For this review, take the finished solid that the model builds, in its own axes (mm). A direction names the side the tool comes from. Coordinates: 2 decimals unless noted, no trailing zeros. Loops run counter-clockwise (first coordinate to the right, second up) from the corner with the lowest first, then second, coordinate; pieces in that order, holes last. Notation, with made-up numbers: M 60,72 L 65,72 A24 ccw 65,101 Z; hole C -12.75,11.5 d5. An arc over 180 degrees is marked long. Answer as a JSON object with one key per item and string values. Group by question number.
Item 1: Insertion check: pin 1 (1 mm diameter, centred on y = 271, z = 5, fed in from +X); pin 2 (4 mm diameter, centred on x = 8.26, y = 258.75, fed in from -Z); pin 3 (1 mm diameter, centred on x = 10.5, z = 1, fed in from -Y) (3 decimals); pin 4 (5 mm diameter, centred on x = -8.26, y = 287.35, fed in from +Z). Each pin has a flat end and moves straight along its axis. Give the tip position at first contact, or say it passes through.
Item 2: Tool access review of faces 4 (the face through (4.5, 273.2, 4.475)), 5 (the face through (-16.783, 270.968, 3.145)): name each direction out of +Z, -Z, +X, -X, +Y, -Y from which nothing blocks a thin tool from reaching the whole face with its end or side.
Item 3: Add section D-D (x = -16.51). State the section outline as (y, z) points (3 decimals), then the cut area to 3 significant figures.
Item 4: Add section C-C (z = 2). State the section outline as (x, y) points (3 decimals), then the cut area to 3 significant figures.
Item 5: Mouldability with a two-part tool opening along Y and no side actions: class faces 1 (the face through (-2.401, 283.863, 1.893)), 2 (the face through (0, 278, 7.015)), 3 (the face through (-4.543, 293.507, 3.458)) as +Y half, -Y half, draft (parallel to the pull), parting line (faces both ways), or undercut.
Item 6: Add section A-A (x = 0). State the section outline as (y, z) points (3 decimals).
Item 7: Add section B-B (y = 273.05). State the section outline as (x, z) points (3 decimals), then the cut area to 3 significant figures.
Item 8: Wall thickness on L1, parallel to Y at x = 0, z = 1.35 (3 decimals); L2, parallel to Y at x = 10, z = 6 (3 decimals); L3, parallel to Y at x = 8, z = 0.75: over which ranges is each line inside the solid? List them lowest first. Write a range as from..to.
Autodesk Inventor part; units mm, degrees
ref_plane "YZ Plane" through (0, 0, 0) normal (1, 0, 0) x (0, 1, 0)
ref_plane "XZ Plane" through (0, 0, 0) normal (0, 1, 0) x (-1, 0, 0)
ref_plane "XY Plane" through (0, 0, 0) normal (0, 0, 1) x (1, 0, 0)
sketch "Sketch1" plane through (0, 0, 0) normal (0, 0, 1) x (1, 0, 0)
  circle A0 centre (0, 273.05) radius 20.955
  circle A1 centre (0, 273.05) radius 11
  arc A2 (219.754, -304.8) -> (225.7704, -296.4188) centre (219.754, -298.45) ccw
  line L0 (225.7704, -296.4188) -> (30.0819, 283.206)
  arc A3 (30.0819, 283.206) -> (-30.0819, 283.206) centre (0, 273.05) ccw
  line L1 (-30.0819, 283.206) -> (-225.7704, -296.4188)
  arc A4 (-225.7704, -296.4188) -> (-219.754, -304.8) centre (-219.754, -298.45) ccw
  line L2 (-219.754, -304.8) -> (219.754, -304.8)
  line L3 (-38.1, -17.4222) -> (-38.1, -222.25)
  arc A5 (-44.45, -228.6) -> (-38.1, -222.25) centre (-44.45, -222.25) ccw
  line L4 (-44.45, -228.6) -> (-113.6024, -228.6)
  arc A6 (-119.6188, -220.2188) -> (-113.6024, -228.6) centre (-113.6024, -222.25) ccw
  line L5 (-119.6188, -220.2188) -> (-50.4664, -15.391)
  arc A7 (-38.1, -17.4222) -> (-50.4664, -15.391) centre (-44.45, -17.4222) ccw
  line L6 (113.6024, -228.6) -> (44.45, -228.6)
  arc A8 (38.1, -222.25) -> (44.45, -228.6) centre (44.45, -222.25) ccw
  line L7 (38.1, -222.25) -> (38.1, -17.4222)
  arc A9 (50.4664, -15.391) -> (38.1, -17.4222) centre (44.45, -17.4222) ccw
  line L8 (50.4664, -15.391) -> (119.6188, -220.2188)
  arc A10 (113.6024, -228.6) -> (119.6188, -220.2188) centre (113.6024, -222.25) ccw
  circle A11 centre (-204.2059, -292.1) radius 2
  circle A12 centre (-187.0552, -241.3) radius 2
  circle A13 centre (187.0552, -241.3) radius 2
  circle A14 centre (204.2059, -292.1) radius 2
  circle A15 centre (19.05, -241.3) radius 2
  circle A16 centre (19.05, -292.1) radius 2
  circle A17 centre (-19.05, -292.1) radius 2
  circle A18 centre (-19.05, -241.3) radius 2
  circle A19 centre (8.255, 287.3481) radius 2
  circle A20 centre (-8.255, 287.3481) radius 2
  circle A21 centre (-16.51, 273.05) radius 2
  circle A22 centre (-8.255, 258.7519) radius 2
  circle A23 centre (8.255, 258.7519) radius 2
  circle A24 centre (16.51, 273.05) radius 2
  circle A25 centre (0, 273.05) radius 11
  circle A26 centre (0, 273.05) radius 11.0762
  circle A27 centre (-8.255, 287.3481) radius 2.1
  circle A28 centre (8.255, 287.3481) radius 2.1
  circle A29 centre (16.51, 273.05) radius 2.1
  circle A30 centre (8.255, 258.7519) radius 2.1
  circle A31 centre (-8.255, 258.7519) radius 2.1
  circle A32 centre (-16.51, 273.05) radius 2.1
  circle A33 centre (0, 273.05) radius 4.35
  point P0 (0, 0)
  dimension "d0" = 0.0762
  dimension "d1" = 4.2
  dimension "d2" = 4.2
  dimension "d3" = 4.2
  dimension "d4" = 4.2
  dimension "d5" = 4.2
  dimension "d6" = 4.2
  dimension "d9" = 8.7
extrude "Extrusion1" add sketch "Sketch1" along normal blind 7.015 contours A0 | A1 | A26
extrude "Extrusion2" cut sketch "Sketch1" along normal blind 4.475 contours A1 | A26 | A33
chamfer "Chamfer1" distance 0.635 angle 45 7 edges at (-11.0762, 273.05, 4.475) (6.155, 287.3481, 7.015) (-10.355, 287.3481, 7.015) (-18.61, 273.05, 7.015) (-10.355, 258.7519, 7.015) (6.155, 258.7519, 7.015) (14.41, 273.05, 7.015)
properties part number "MainOuterBearingMount"
From the geometry:
{
 "1": {"pin 1": "stops at x = 20.9", "pin 2": "passes through", "pin 3": "stops at y = 254.635", "pin 4": "stops at z = 6.79"},
 "2": {"face 4": "-Z", "face 5": "+Z, -Z"},
 "3": {"outline": "M 260.145,0 L 270.95,0 L 270.95,6.38 L 270.315,7.015 L 260.145,7.015 Z; M 275.15,0 L 285.955,0 L 285.955,7.015 L 275.785,7.015 L 275.15,6.38 Z", "area": "151 mm²"},
 "4": {"outline": "C 0,273.05 d41.91; hole C -16.51,273.05 d4.2; hole C 0,273.05 d22.152; hole C -8.255,258.752 d4.2; hole C -8.255,287.348 d4.2; hole C 8.255,258.752 d4.2; hole C 8.255,287.348 d4.2; hole C 16.51,273.05 d4.2", "area": "911 mm²"},
 "5": {"face 1": "undercut", "face 2": "draft", "face 3": "parting line"},
 "6": {"outline": "M 252.095,0 L 261.974,0 L 261.974,3.84 L 262.609,4.475 L 268.7,4.475 L 268.7,7.015 L 252.095,7.015 Z; M 277.4,4.475 L 283.491,4.475 L 284.126,3.84 L 284.126,0 L 294.005,0 L 294.005,7.015 L 277.4,7.015 Z"},
 "7": {"outline": "M -20.955,0 L -18.61,0 L -18.61,6.38 L -19.245,7.015 L -20.955,7.015 Z; M -14.41,0 L -11.076,0 L -11.076,3.84 L -10.441,4.475 L -4.35,4.475 L -4.35,7.015 L -13.775,7.015 L -14.41,6.38 Z; M 4.35,4.475 L 10.441,4.475 L 11.076,3.84 L 11.076,0 L 14.41,0 L 14.41,6.38 L 13.775,7.015 L 4.35,7.015 Z; M 18.61,0 L 20.955,0 L 20.955,7.015 L 19.245,7.015 L 18.61,6.38 Z", "area": "113 mm²"},
 "8": {"L1": "y = 252.095..261.974, 284.126..294.005", "L2": "y = 254.635..257.584, 259.92..286.18, 288.516..291.465", "L3": "y = 253.68..256.67, 260.84..265.39, 280.71..285.26, 289.43..292.42"}
}
